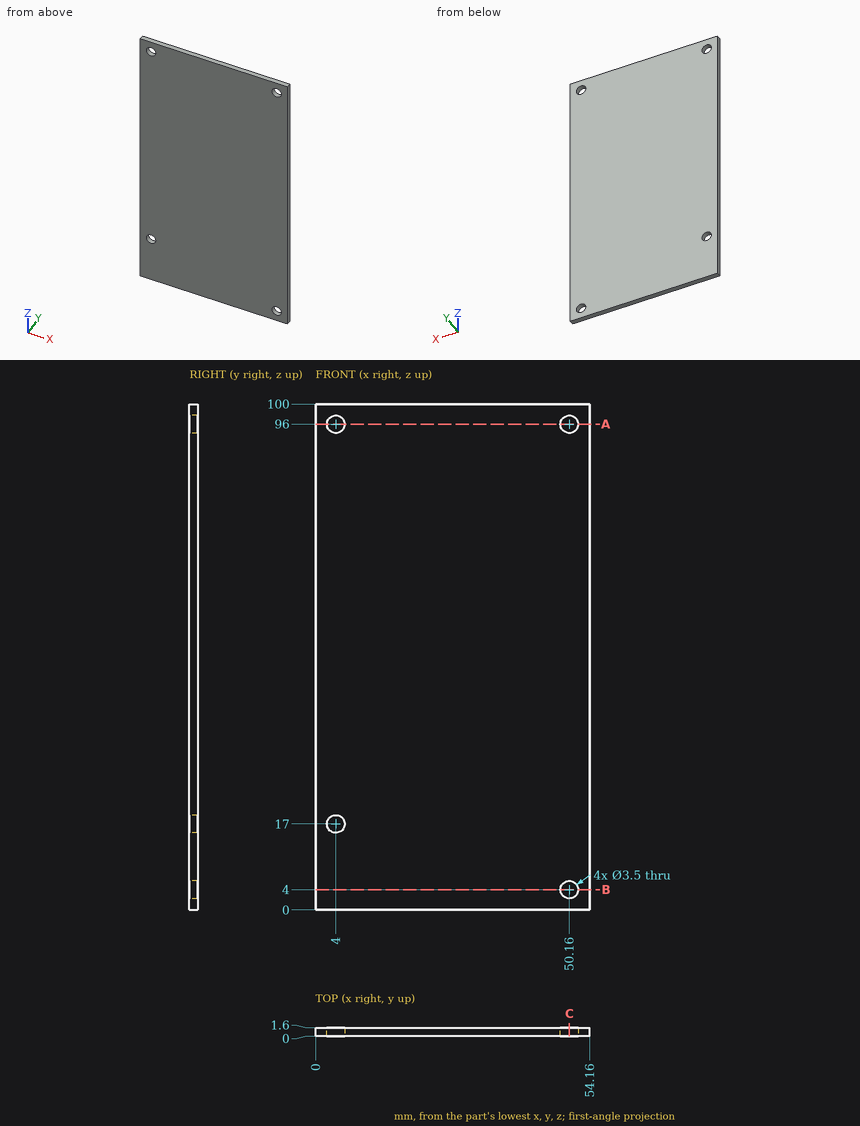
Verification items for this drawing (mm, ordinates from the low corner). Give positions to 0.01 mm unless a question says otherwise; leave off trailing zeros. Loops run counter-clockwise (first coordinate to the right, second up) from the corner with the lowest first, then second, coordinate; pieces in that order, holes last.
(1) Depth check by flat-ended pin: pin 1 Ø3 at (x, z) = (50.16, 96) entering from +Y. Enter the tip coordinate at first touch or a pass-through.
From the geometry:
pin 1: passes through
(2) Section check B-B on z = 4. Record the cut outline in (x, y), then the cut area to 3 significant figures.
From the geometry:
outline: (0, 0) - (48.41, 0) - (48.41, 1.6) - (0, 1.6) - close; (51.91, 0) - (54.16, 0) - (54.16, 1.6) - (51.91, 1.6) - close
area: 81.1 mm2
(3) Section check A-A on z = 96. Record the cut outline in (x, y).
From the geometry:
outline: (0, 0) - (2.25, 0) - (2.25, 1.6) - (0, 1.6) - close; (5.75, 0) - (48.41, 0) - (48.41, 1.6) - (5.75, 1.6) - close; (51.91, 0) - (54.16, 0) - (54.16, 1.6) - (51.91, 1.6) - close
(4) Section check C-C on x = 50.16. Record the cut outline in (y, z), then the cut area to 3 significant figures.
From the geometry:
outline: (0, 0) - (1.6, 0) - (1.6, 2.25) - (0, 2.25) - close; (0, 5.75) - (1.6, 5.75) - (1.6, 94.25) - (0, 94.25) - close; (0, 97.75) - (1.6, 97.75) - (1.6, 100) - (0, 100) - close
area: 149 mm2
(5) Thickness scan on L1, parallel to Z at x = 50.16, y = 0.9; L2, parallel to Z at x = 4, y = 1.25; L3, parallel to X at y = 0.6, z = 96. Record the ranges inside material, lowest first.
From the geometry:
L1: z = 0 to 2.25, 5.75 to 94.25, 97.75 to 100
L2: z = 0 to 15.25, 18.75 to 94.25, 97.75 to 100
L3: x = 0 to 2.25, 5.75 to 48.41, 51.91 to 54.16
